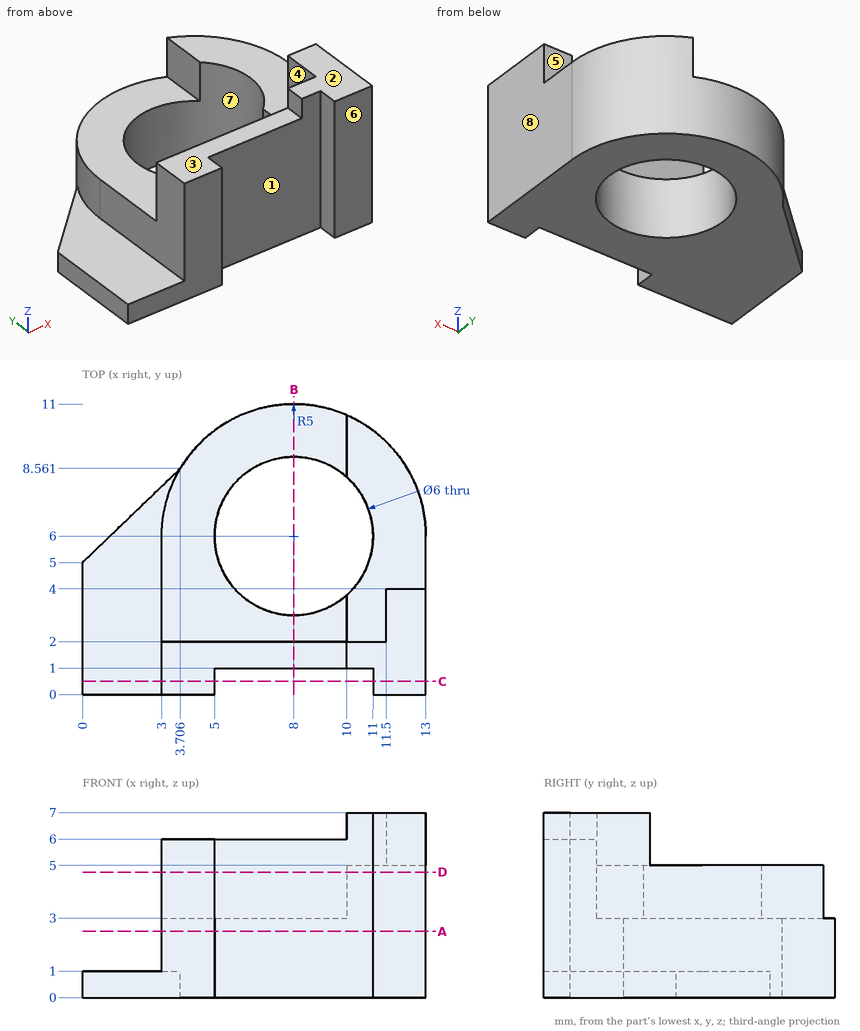
Could you check a few things on this drawing? It's one solid part, dimensions in mm from its lowest x, y, z. A direction names the side the tool comes from. Coordinates: 2 decimals unless noted, no trailing zeros. Order: outer loops, then holes, each group sorted by start corner. A loop starts at its lowest first (then second) coordinate and runs counter-clockwise, first axis right, second up. Notation, with made-up numbers: (44, -18.75) -> (79, -18.75) arc R19 ccw to (79, -2.75) -> close; hole circle Ø11 at (54.5, 44). An arc over 180 degrees is marked (long way). One line per item, written item: value. Start each with the question number.
1) If I drill on L1, parallel to Y at x = 8, z = 3.4; L2, parallel to X at y = 2.25, z = 2; L3, parallel to Y at x = 8, z = 2.75, over which ranges is the centre line in solid material (lowest first)? Write a range as [from, to].
2) Imagine slicing it at B-B on x = 8. List the corners of the cut face in (y, z) for me.
3) Which directions (+Z, -Z, +X, -X, +Y, -Y) give clear straight access to the entire face, cutting with the end or side of a thin tool? Please do the marked faces 1, 2, 3, 4 and 5.
4) Imagine slicing it at A-A on z = 2.5. List the corners of the cut face in (x, y) for me, plus the area to 3 significant figures.
5) I'm going to push flat-ended pins straight in: pin 1 (3.5 mm diameter, centred on x = 8, y = 6, fed in from +Z); pin 2 (0.8 mm diameter, centred on y = 0.5, z = 2.5, fed in from -X); pin 3 (0.8 mm diameter, centred on y = 1.5, z = 6.5, fed in from -X); pin 4 (1 mm diameter, centred on y = 3, z = 6.5, fed in from -X). Where does each tip first touch, or does it pass through?
6) Imagine slicing it at D-D on z = 4.75. List the corners of the cut face in (x, y) for me, plus the area to 3 significant figures.
7) Imagine slicing it at C-C on y = 0.5. List the corners of the cut face in (x, z) for me, plus the area to 3 significant figures.
8) We'd pull the mould along Y, two halves only. Please class the marked faces 6, 7 and 8: +Y half, -Y half, draft (parallel to the pull), parting line (faces both ways), or undercut.
Answer list:
1. L1: y = [1, 2]
1. L2: x = [3, 13]
1. L3: y = [1, 3], [9, 11]
2. outline: (1, 0) -> (3, 0) -> (3, 3) -> (2, 3) -> (2, 6) -> (1, 6) -> close; (9, 0) -> (11, 0) -> (11, 3) -> (9, 3) -> close
3. face 1: +Z, -Z, -Y
3. face 2: +Z, +X, -X, +Y, -Y
3. face 3: +Z, -X, +Y, -Y
3. face 4: +Z, -X, +Y
3. face 5: +Z, +X, -X, +Y
4. outline: (3, 0) -> (5, 0) -> (5, 1) -> (11, 1) -> (11, 0) -> (13, 0) -> (13, 6) arc R5 ccw to (3, 6) -> close; hole circle Ø6 at (8, 6)
4. area: 65.0 mm2
5. pin 1: passes through
5. pin 2: stops at x = 3
5. pin 3: stops at x = 10
5. pin 4: stops at x = 11.5
6. outline: (3, 0) -> (5, 0) -> (5, 1) -> (11, 1) -> (11, 0) -> (13, 0) -> (13, 6) arc R5 ccw to (10, 10.58) -> (10, 8.24) arc R3 cw to (10, 3.76) -> (10, 2) -> (3, 2) -> close
6. area: 32.8 mm2
7. outline: (0, 0) -> (5, 0) -> (5, 6) -> (3, 6) -> (3, 1) -> (0, 1) -> close; (11, 0) -> (13, 0) -> (13, 7) -> (11, 7) -> close
7. area: 29.0 mm2
8. face 6: -Y half
8. face 7: undercut
8. face 8: draft
